Design review of the part built by this model. Coordinates are the model's own, in mm. A direction names the side the tool comes from. Give positions to 0.01 mm unless a question says otherwise; leave off trailing zeros. Write each loop counter-clockwise with the first axis right and the second up, starting at its lowest first coordinate (ties: lowest second). Pieces come first, ordered by that corner, then holes. Notation, with made-up numbers: (77, 49) -> (102, 49) arc R28 ccw to (102, 87) -> close; hole circle Ø3 at (73.25, 3.5). An arc over 180 degrees is marked (long way). Answer as a JSON object with one key per item and string values.
```python
from build123d import *

# Parameters (mm, degrees)
BOSS_EXTRUDE1_DEPTH = 6.35


with BuildPart() as part:
    # Sketch1 → Boss-Extrude1 (new body)
    with BuildSketch(Plane(origin=(0, 0, 0), x_dir=(0, 0, -1), z_dir=(1, 0, 0))):
        with BuildLine():
            Line((-6.35, 12.7), (1.833087105, 12.7))
            Line((1.833087105, 12.7), (6.751108029, 21.218262114))
            ThreePointArc((6.751108029, 21.218262114), (19.7625, 34.229654085), (15, 16.455762114))
            Line((15, 16.455762114), (6.35, 1.473522628))
            Line((6.35, 1.473522628), (6.35, -12.7))
            Line((6.35, -12.7), (-6.35, -12.7))
            Line((-6.35, -12.7), (-6.35, 12.7))
        make_face()
    extrude(amount=BOSS_EXTRUDE1_DEPTH)


solid = part.part
```
(1) We need section A-A, the plane x = 4.25. State the section outline as (y, z) points (3 decimals).
Here are the results:
{"outline": "(-12.7, -6.35) -> (1.474, -6.35) -> (16.456, -15) arc R9.525 ccw (long way) to (21.218, -6.751) -> (12.7, -1.833) -> (12.7, 6.35) -> (-12.7, 6.35) -> close"}
(2) For faces 1 (the flat face through (3.13, 16.9, -4.26)), 2 (the flat face through (3, -6, -6.35)), 3 (the flat face through (3, 12.7, 2)), 4 (the cylindrical face through (3.131, 34.399, -19.457)), 5 (the flat face through (6.35, 12, -6)), list the 3-axis set-ups (+Z, -Z, +X, -X, +Y, -Y) from which the entire face can be reached by the end or side of a thin tool; tool diameter is ignored.
Here are the results:
{"face 1": "+Z, +X, -X", "face 2": "-Z, +X, -X, -Y", "face 3": "+Z, +X, -X, +Y", "face 4": "+X, -X", "face 5": "+Z, -Z, +X, +Y, -Y"}
(3) We need section B-B, the plane y = -2.5. State the section outline as (x, z) points, then the cut area to 3 significant figures.
Here are the results:
{"outline": "(0, -6.35) -> (6.35, -6.35) -> (6.35, 6.35) -> (0, 6.35) -> close", "area": "80.6 mm²"}
(4) For line 1 along Z through (x, y) = (3.5, -2); line 2 along Y through (x, z) = (0.5, -1); line 3 along Z through (x, y) = (4, 9), list the stretches that pass through material, from the lowest coordinate up.
Here are the results:
{"line 1": "z = -6.35 to 6.35", "line 2": "y = -12.7 to 12.7", "line 3": "z = -10.7 to 6.35"}
(5) Clearance check with flat-ended pins moving along their axes: pin 1 (3 mm diameter, centred on x = 1, y = 17, fed in from +Z); pin 2 (2 mm diameter, centred on x = 1.5, y = 14, fed in from +Z); pin 3 (3 mm diameter, centred on x = 3.5, y = 14.5, fed in from -Z). State where each tip first meets the part, or that it passes through.
Here are the results:
{"pin 1": "stops at z = -3.45", "pin 2": "stops at z = -2.01", "pin 3": "stops at z = -14.74"}
(6) We need section C-C, the plane z = -18. State the section outline as (x, y) points, then the cut area to 3 significant figures.
Here are the results:
{"outline": "(0, 16.94) -> (6.35, 16.94) -> (6.35, 35.02) -> (0, 35.02) -> close", "area": "115 mm²"}
